The listing builds one solid part. Answer for the finished solid, in the listing's coordinates (mm). A direction names the side the tool comes from. Round coordinates to 2 decimals unless told otherwise and drop trailing zeros. Write each loop counter-clockwise with the first axis right and the second up, starting at its lowest first coordinate (ties: lowest second). Pieces come first, ordered by that corner, then holes. Notation, with made-up numbers: M 1.5,-37.75 L 30.5,-37.75 A33 cw 30.5,-9.75 Z; hole C -33,2.5 d1. An arc over 180 degrees is marked long. Write each question's results on one line, items separated by ' | '.
from build123d import *

# Parameters (mm, degrees)
F0_R     = 13
F1_DEPTH = 10
F2_SIZE  = 4
F3_SIZE  = 4
F5_D     = 5
F5_DEPTH = 8
F5_TIP   = 1.5021515476


with BuildPart() as f1:
    # F0 (on Front) → F1 (new body)
    with BuildSketch(Plane.XZ):
        Polygon((-10, 0), (0, 0), (10, 0), (10, -10), (30, -10), (30, 0), (50, 0), (50, -10), (70, -10), (70, 0), (90, 0), (90, 15), (70, 15), (21, 258), (21, 300), (0, 300), (-21, 300), (-21, 258), (-70, 15), (-90, 15), (-90, 0), (-70, 0), (-70, -10), (-50, -10), (-50, 0), (-30, 0), (-30, -10), (-10, -10), align=None)
        with BuildLine():
            ThreePointArc((7.5, 50), (0, 42.5), (-7.5, 50))
            Line((-7.5, 50), (-7.5, 199.0483840028))
            ThreePointArc((-7.5, 199.0483840028), (0, 207.5601304887), (7.5, 199.0483840028))
            Line((7.5, 199.0483840028), (7.5, 50))
        make_face(mode=Mode.SUBTRACT)
        with Locations((0, 279)):
            Circle(F0_R, mode=Mode.SUBTRACT)
    extrude(amount=F1_DEPTH)

    # F2
    f2_edges = [f1.edges().sort_by_distance(p)[0] for p in [
        (21, -5, 300),
        (-21, -5, 300),
    ]]
    chamfer(f2_edges, length=F2_SIZE)

    # F3
    f3_edges = [f1.edges().sort_by_distance(p)[0] for p in [
        (-90, -5, 15),
        (90, -5, 15),
    ]]
    chamfer(f3_edges, length=F3_SIZE)

    # F5
    with Locations(Plane(origin=(0, 0, 0), x_dir=(1, 0, 0), z_dir=(0, 0, -1))):
        with Locations((-80, 5), (80, 5)):
            Hole(F5_D / 2, depth=F5_DEPTH)
            with Locations((0, 0, -(F5_DEPTH + F5_TIP / 2))):  # 118° drill point
                Cone(0, F5_D / 2, F5_TIP, mode=Mode.SUBTRACT)


solid = f1.part
1) Section C-C (z = 144.5) is taken. Determine the outline of the cut face in (x, y), then the cut area to 3 significant figures.
Return value:
outline: M -43.89,-10 L -7.5,-10 L -7.5,0 L -43.89,0 Z; M 7.5,-10 L 43.89,-10 L 43.89,0 L 7.5,0 Z | area: 728 mm²
2) Find the intervals of material crossed by line 1 (Z direction, x = 0, y = -4.5); line 2 (Z direction, x = -6, y = -9.5); line 3 (Y direction, x = 80, z = 3), in increasing order.
Return value:
line 1: 0 to 42.5, 207.56 to 266, 292 to 300 | line 2: 0 to 45.5, 204.6 to 267.47, 290.53 to 300 | line 3: -10 to -7.5, -2.5 to 0
3) The mould has two halves that part along Z. Classify faces 4 (the face through (40, -5, 0)), 5 (the face through (-0.18, -4.93, 207.558)), 6 (the face through (19, -10, 113)): +Z half, -Z half, draft (parallel to the pull), parting line (faces both ways), or undercut.
Return value:
face 4: -Z half | face 5: undercut | face 6: draft
4) A tool of negligible diameter and unlimited length cuts with its end or side. For faces 1 (the face through (7.5, -5, 126)), 2 (the face through (-82.4, -3.8, 0)), 3 (the face through (-30, -5, -5)), from which of +Z, -Z, +X, -X, +Y, -Y can it reach the whole face along a straight path? Write none if from no direction.
Return value:
face 1: +Y, -Y | face 2: -Z, -X, +Y, -Y | face 3: -Z, +Y, -Y
5) Each of these flat-tipped pins is pushed along its axis until it touches: pin 1 (3 mm diameter, centred on y = -5.5, z = -2.5, fed in from -X); pin 2 (3 mm diameter, centred on x = -43.5, y = -5, fed in from -Z); pin 3 (5 mm diameter, centred on x = -80.5, y = -6, fed in from +Z). Where does it stop, or does it pass through?
Return value:
pin 1: x = -70 | pin 2: z = 0 | pin 3: z = 15
6) Section D-D (x = -40.5) is taken. Determine the outline of the cut face in (y, z), then the cut area to 3 significant figures.
Return value:
outline: M -10,0 L 0,0 L 0,161.3 L -10,161.3 Z | area: 1,610 mm²
7) Section A-A (x = 0) is taken. Determine the outline of the cut face in (y, z).
Return value:
outline: M -10,0 L 0,0 L 0,42.5 L -10,42.5 Z; M -10,207.56 L 0,207.56 L 0,266 L -10,266 Z; M -10,292 L 0,292 L 0,300 L -10,300 Z
8) Section B-B (z = 279) is taken. Determine the outline of the cut face in (x, y).
Return value:
outline: M -21,-10 L -13,-10 L -13,0 L -21,0 Z; M 13,-10 L 21,-10 L 21,0 L 13,0 Z
